Verification items for the finished model (mm, model axes). A direction names the side the tool comes from. Round coordinates to 2 decimals unless told otherwise and drop trailing zeros. Write each loop counter-clockwise with the first axis right and the second up, starting at its lowest first coordinate (ties: lowest second). Pieces come first, ordered by that corner, then holes. Notation, with made-up numbers: M -27,-20 L -23,-20 A8 ccw -23,-16 Z; hole C -3,37 d5. An arc over 180 degrees is marked long. Use a Markdown table: item, result. Add a question column.
from build123d import *

# Parameters (mm, degrees)
SKETCH_W        = 7
SKETCH_H        = 7
SKETCH_R        = 1.55
PAD_DEPTH       = 33.7
SKETCH001_W     = 3.5
SKETCH001_H     = 9.1
POCKET_DEPTH    = 7.001
POCKET_FACE10_W = 33.7
POCKET_FACE10_H = 7
PAD001_DEPTH    = 1
CHAMFER_SIZE    = 1.5


with BuildPart() as part:
    # Sketch → Pad (new body)
    with BuildSketch(Plane.XZ):
        Rectangle(SKETCH_W, SKETCH_H)
        Circle(SKETCH_R, mode=Mode.SUBTRACT)
    extrude(amount=PAD_DEPTH)

    # Sketch001 (on Face2 of Pad) → Pocket (cut, through all)
    with BuildSketch(Plane(origin=(0, 0, -3.5), x_dir=(1, 0, 0), z_dir=(0, 0, -1))):
        with Locations((-1.75, 29.15)):
            Rectangle(SKETCH001_W, SKETCH001_H)
        with Locations((-1.75, 4.55)):
            Rectangle(SKETCH001_W, SKETCH001_H)
    extrude(amount=-POCKET_DEPTH, mode=Mode.SUBTRACT)

    # Pocket Face10 → Pad001 (add)
    with BuildSketch(Plane(origin=(3.5, -16.85, 0), x_dir=(0, -1, 0), z_dir=(1, 0, 0))):
        Rectangle(POCKET_FACE10_W, POCKET_FACE10_H)
    extrude(amount=PAD001_DEPTH)

    # Chamfer
    chamfer_edges = [part.edges().sort_by_distance(p)[0] for p in [
        (-3.5, -24.6, 0),
        (-3.5, -9.1, 0),
    ]]
    chamfer(chamfer_edges, length=CHAMFER_SIZE)


solid = part.part
1. Access from +Z, -Z, +X, -X, +Y, -Y to the whole of each face (thin tool, end or side, straight path). Record for faces 5 (the flat face through (0, -4, 3)), 6 (the flat face through (-1.5, -24.6, -0.8)), 7 (the flat face through (-3.5, -17, 0)).
2. Cross-section at A-A on z = 0. Enter the section's corners in (x, y).
3. Depth check by flat-ended pin: pin 1 Ø2 at (y, z) = (-6, 2) entering from -X; pin 2 Ø2 at (x, z) = (-1, 0.5) entering from +Y; pin 3 Ø1 at (x, z) = (0.5, -2) entering from +Y; pin 4 Ø3 at (x, z) = (0, 0) entering from -Y. Enter the tip coordinate at first touch or a pass-through.
4. Cross-section at B-B on x = -1.25. Enter the section's corners in (y, z).
5. Cross-section at D-D on y = -22. Enter the section's corners in (x, z), plus the area to 3 significant figures.
6. Release check for a two-part mould opening along X. For faces 1 (the flat face through (-1.5, -9.1, -0.8)), 2 (the flat face through (4.5, -17, 0)), 3 (the cylindrical face through (1.478, -16.614, 0.466)), 4 (the flat face through (0, -29, 3)) record: +X half, -X half, draft (parallel to the pull), parting line (faces both ways), or undercut.
7. Scan lines: line 1 along Z through (x, y) = (0, -18.5); line 2 along X through (y, z) = (-20.5, 0); line 3 along X through (y, z) = (-9, -3). Record each from-to range of solid material in increasing order. Write a range as from..to.
8. Cross-section at C-C on y = -29.5. Enter the section's corners in (x, z).
Answer:
| question | item | result |
|---|---|---|
| 1 | face 5 | +Z, -Z, -X, +Y |
| 1 | face 6 | +Z, -Z, -X, -Y |
| 1 | face 7 | +Z, -Z, -X, +Y, -Y |
| 2 | outline | M -3.5,-23.1 L -2,-24.6 L -1.55,-24.6 L -1.55,-9.1 L -2,-9.1 L -3.5,-10.6 Z; M 1.55,-33.7 L 4.5,-33.7 L 4.5,0 L 1.55,0 Z |
| 3 | pin 1 | stops at x = 0 |
| 3 | pin 2 | stops at y = -9.1 |
| 3 | pin 3 | stops at y = 0 |
| 3 | pin 4 | passes through |
| 4 | outline | M -24.6,-3.5 L -9.1,-3.5 L -9.1,-0.92 L -24.6,-0.92 Z; M -24.6,0.92 L -9.1,0.92 L -9.1,3.5 L -24.6,3.5 Z |
| 5 | outline | M -3.5,-3.5 L 4.5,-3.5 L 4.5,3.5 L -3.5,3.5 Z; hole C 0,0 d3.1 |
| 5 | area | 48.5 mm^2 |
| 6 | face 1 | draft |
| 6 | face 2 | +X half |
| 6 | face 3 | undercut |
| 6 | face 4 | -X half |
| 7 | line 1 | z = -3.5..-1.55, 1.55..3.5 |
| 7 | line 2 | x = -3.5..-1.55, 1.55..4.5 |
| 7 | line 3 | x = 0..4.5 |
| 8 | outline | M 0,-3.5 L 4.5,-3.5 L 4.5,3.5 L 0,3.5 L 0,1.55 A1.55 cw 0,-1.55 Z |
